from build123d import *

# Parameters (mm, degrees)
F5_W      = 8.89
F5_H      = 8.89
F6_DEPTH  = 57.15
F6_FACE_W = 8.89
F6_FACE_H = 8.89
F7_DEPTH  = 0.254
F9_DEPTH  = 57.15
F10_SIZE  = 6.35
F11_SIZE  = 6.35


with BuildPart() as f3:
    # F2 (on offset) → F3 section 0
    with BuildSketch(Plane.XZ.offset(114.3)):
        Polygon((0.508, 13.208), (0, 13.208), (0, -12.192), (0, -12.7), (76.2, -12.7), (76.2, -12.192), (76.2, 13.208), (75.692, 13.208), (75.692, -12.192), (0.508, -12.192), align=None)
    # F0 (on Front) → F3 section 1
    with BuildSketch(Plane.XZ):
        Polygon((0.508, 0), (0, 0), (0, -24.892), (0, -25.4), (51.816, -25.4), (51.816, -24.892), (51.816, 0), (51.308, 0), (51.308, -24.892), (0.508, -24.892), align=None)
    loft()

    # F5 (on face) → F6 (join)
    with BuildSketch(Plane.XY.offset(-12.192)):
        with Locations((8.128, -109.855)):
            Rectangle(F5_W, F5_H)
    extrude(amount=F6_DEPTH)

    # F6_face (on face) → F7 (join)
    with BuildSketch(Plane(origin=(8.128, -109.855, -12.192), x_dir=(1, 0, 0), z_dir=(0, 0, -1))):
        Rectangle(F6_FACE_W, F6_FACE_H)
    extrude(amount=F7_DEPTH)

    # F8 (on face) → F9 (join)
    with BuildSketch(Plane.YZ.offset(12.573)):
        with BuildLine():
            Line((-112.014, 19.304), (-114.3, 19.304))
            Line((-114.3, 19.304), (-114.3, -12.192))
            add(Edge.make_bspline(
                [(-114.3, -12.192), (-113.728496, -12.2555), (-113.156994, -12.319001), (-112.585496, -12.3825), (-112.014, -12.446)],
                knots=[0, 0, 0, 0, 0, 1, 1, 1, 1, 1], degree=4))
            Line((-112.014, -12.446), (-112.014, 19.304))
        make_face()
    extrude(amount=F9_DEPTH)

    # F10
    f10_edges = [f3.edges().sort_by_distance(p)[0] for p in [
        (3.683, -109.855, 44.958),
    ]]
    chamfer(f10_edges, length=F10_SIZE)

    # F11
    f11_edges = [f3.edges().sort_by_distance(p)[0] for p in [
        (11.303, -105.41, 44.958),
    ]]
    chamfer(f11_edges, length=F11_SIZE)


solid = f3.part
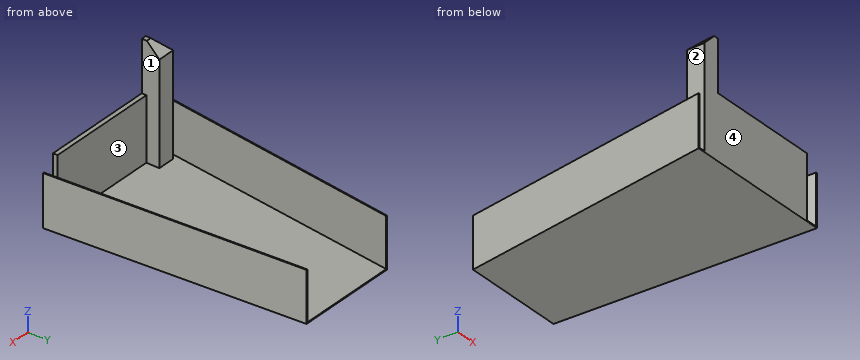
The model under review builds one solid part; all positions refer to its coordinate system, in mm. Face numbers are marked on the shaded views. A direction names the side the tool comes from. Coordinates: 2 decimals unless noted, no trailing zeros. Write each loop counter-clockwise with the first axis right and the second up, starting at its lowest first coordinate (ties: lowest second). Pieces come first, ordered by that corner, then holes. Notation, with made-up numbers: M 21.5,-11 L 45.5,-11 A20 ccw 45.5,23 Z; hole C 75,63 d4. An arc over 180 degrees is marked long. Put each result on its own line as item: value.
1) Add section B-B on z = 18. Give the boundary of the cut face in (x, y).
Computed:
outline: M 3.68,-114.3 L 69.72,-114.3 L 69.72,-112.01 L 12.57,-112.01 L 12.57,-105.41 L 3.68,-105.41 Z
2) Clearance check with flat-ended pins moving along their axes: pin 1 Ø10 at (x, y) = (30.5, -37) entering from -Z; pin 2 Ø5.5 at (x, y) = (8.5, -108) entering from -Z; pin 3 Ø2.5 at (y, z) = (-110, 25.5) entering from -X; pin 4 Ø1.8 at (y, z) = (-113.5, 10.5) entering from +X. State where each tip first meets the part, or that it passes through.
Computed:
pin 1: stops at z = -21.84
pin 2: stops at z = -13.71
pin 3: stops at x = 3.68
pin 4: stops at x = 76.2
3) Wall thickness on probe 1 along Y at (x, z) = (68, 17); probe 2 along X at (y, z) = (-107.5, 16); probe 3 along Y at (x, z) = (5, -5.5): over which ranges is each line inside the solid? List them lowest first. Write a range as [from, to].
Computed:
probe 1: y = [-114.3, -112.01]
probe 2: x = [3.68, 12.57]
probe 3: y = [-114.3, -105.41]
4) Draft analysis for pull direction X (two halves, no side actions). For the marked faces 3 and 4, state which applies: released by +X, released by -X, zero draft, split by the parting line, or undercut.
Computed:
face 3: undercut
face 4: zero draft
5) Add section A-A on z = -10.5. State how many separate pieces and enclosed holes the cut face has, then the cut area to 3 significant figures.
Computed:
separate pieces: 3
enclosed holes: 0
area: 326 mm2
6) For the marked faces 1 and 2, list the 3-axis set-ups (+Z, -Z, +X, -X, +Y, -Y) from which the entire face can be reached by the end or side of a thin tool; tool diameter is ignored.
Computed:
face 1: +Z, +Y
face 2: +Z, +Y, -Y
7) Add section D-D on z = 36. Give the boundary of the cut face in (x, y), then the cut area to 3 significant figures.
Computed:
outline: M 3.68,-114.3 L 12.57,-114.3 L 12.57,-105.41 L 3.68,-105.41 Z
area: 79.0 mm2
